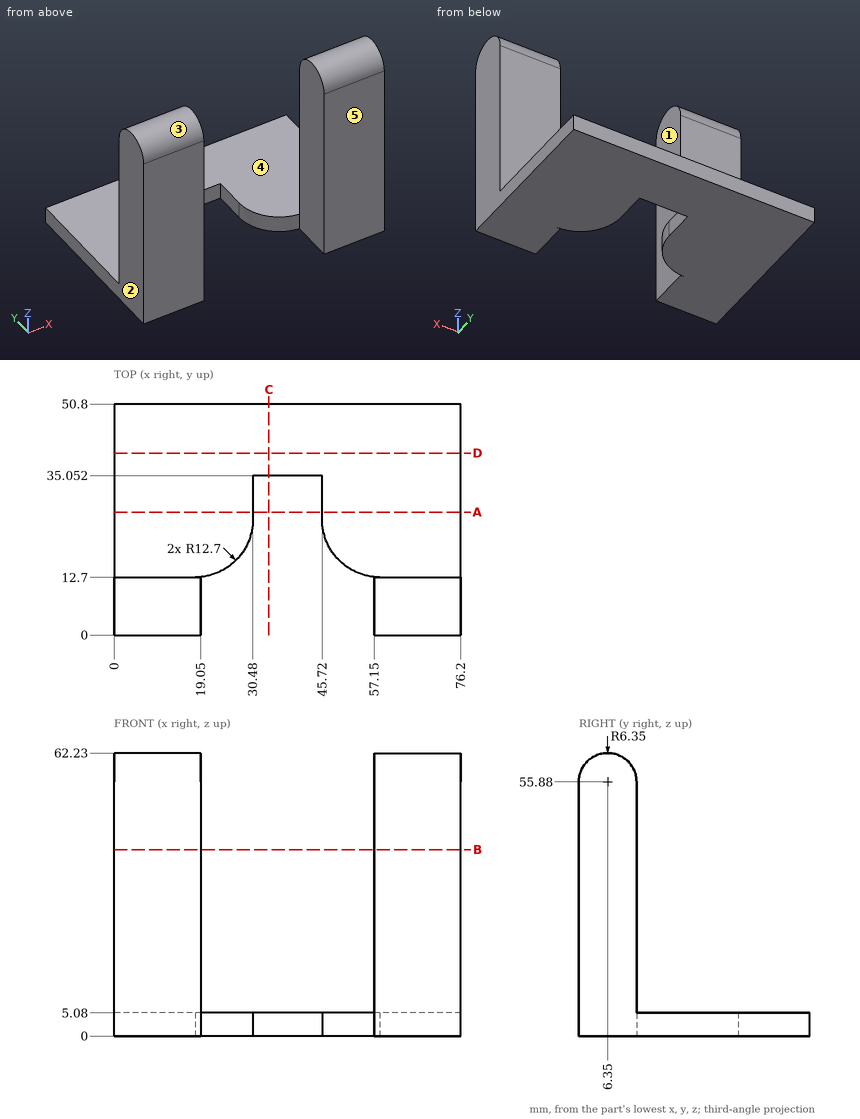
Can you work these out from the drawing? Everything is in mm from the part's minimum corner. A direction names the side the tool comes from. Coordinates: 2 decimals unless noted, no trailing zeros. Loops run counter-clockwise (first coordinate to the right, second up) from the corner with the lowest first, then second, coordinate; pieces in that order, holes last. Notation, with made-up numbers: M 44.25,59.5 L 70.25,59.5 A20 cw 70.25,86.5 Z; hole C 54.5,21 d3. An arc over 180 degrees is marked long. Put each result on its own line as item: value. Start each with the question number.
(1) Suppose I cut it at B-B on z = 41. Please give me the cut outline in (x, y), then the cut area to 3 significant figures.
(2) Suppose I cut it at D-D on y = 40. Please give me the cut outline in (x, z).
(3) Thinking about a two-plate mould opening in X: for the marked faces 1, 2 and 3, which applies, pulls with the +X half, pulls with the -X half, needs draft (parallel to the pull), parting line crosses it, or undercut?
(4) Suppose I cut it at A-A on y = 27. Please give me the cut outline in (x, z), then the cut area to 3 significant figures.
(5) For the marked faces 4 and 5, which set-ups out of +Z, -Z, +X, -X, +Y, -Y let a thin tool reach every point of the face, with its end or its side?
(6) I need wall thicknesses on line 1 (X direction, y = 6, z = 34); line 2 (Y direction, x = 5, z = 7.5); line 3 (Z direction, x = 13.5, y = 38). Which ranges of each line are inside material? Lowest first, please. Write a range as from..to.
(7) Will these pins go through, and if not, where does the flat tip stop? P1, Ø5.5, axis at x = 14, z = 32, coming from the +Y side; P2, Ø19, axis at x = 33, y = 33, coming from the +Z side; P3, Ø2.5, axis at x = 39, z = 2, coming from the -Y side.
(8) Suppose I cut it at C-C on x = 34. Please give me the cut outline in (y, z), then the cut area to 3 significant figures.
Solutions:
1. outline: M 0,0 L 19.05,0 L 19.05,12.7 L 0,12.7 Z; M 57.15,0 L 76.2,0 L 76.2,12.7 L 57.15,12.7 Z
1. area: 484 mm2
2. outline: M 0,0 L 76.2,0 L 76.2,5.08 L 0,5.08 Z
3. face 1: undercut
3. face 2: pulls with the -X half
3. face 3: needs draft
4. outline: M 0,0 L 30.48,0 L 30.48,5.08 L 0,5.08 Z; M 45.72,0 L 76.2,0 L 76.2,5.08 L 45.72,5.08 Z
4. area: 310 mm2
5. face 4: +Z, +X, -X, +Y
5. face 5: +Z, -Z, +X, -X, -Y
6. line 1: x = 0..19.05, 57.15..76.2
6. line 2: y = 0..12.7
6. line 3: z = 0..5.08
7. P1: stops at y = 12.7
7. P2: stops at z = 5.08
7. P3: stops at y = 35.05
8. outline: M 35.05,0 L 50.8,0 L 50.8,5.08 L 35.05,5.08 Z
8. area: 80.0 mm2
